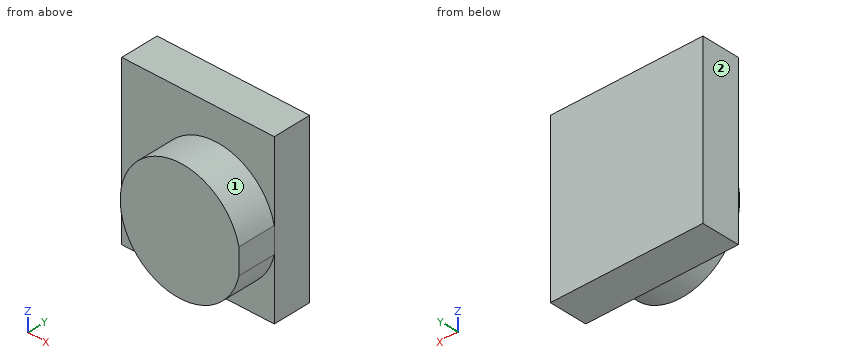
from build123d import *

# Parameters (mm, degrees)
F0_W     = 101.685505
F0_H     = 110.430561
F1_DEPTH = 25.4
F3_DEPTH = 25.4


with BuildPart() as f1:
    # F0 (on Front) → F1 (new body)
    with BuildSketch(Plane.XZ):
        with Locations((-2.378846, 5.691071)):
            Rectangle(F0_W, F0_H)
    extrude(amount=F1_DEPTH)

    # F2 (on face) → F3 (join)
    with BuildSketch(Plane.XZ.offset(25.4)):
        with BuildLine():
            Line((48.463907, -8.572468), (48.463907, 8.572468))
            ThreePointArc((48.463907, 8.572468), (-30.630272, 0), (48.463907, -8.572468))
        make_face()
    extrude(amount=F3_DEPTH)


solid = f1.part
The model under review builds one solid part; all positions refer to its coordinate system, in mm. Face numbers are marked on the shaded views. A direction names the side the tool comes from. Give positions to 0.01 mm unless a question says otherwise; leave off trailing zeros. Loops run counter-clockwise (first coordinate to the right, second up) from the corner with the lowest first, then second, coordinate; pieces in that order, holes last. Notation, with made-up numbers: (47, 0) -> (101, 0) arc R11 cw to (101, 9) -> close; hole circle Ø11 at (47, 31). An arc over 180 degrees is marked (long way). Put each result on its own line as item: value. Start each with the question number.
1. We need section C-C on y = -31.5. State the section outline as (x, z) points, then the cut area to 3 significant figures.
2. Wall thickness on probe 1 along Y at (x, z) = (43.5, 56); probe 2 along Z at (x, y) = (27, -41); probe 3 along X at (y, z) = (-28.5, 34.5): over which ranges is each line inside the solid? List them lowest first.
3. We need section B-B on x = 20. State the section outline as (y, z) points.
4. For the marked faces 1 and 2, list the 3-axis set-ups (+Z, -Z, +X, -X, +Y, -Y) from which the entire face can be reached by the end or side of a thin tool; tool diameter is ignored.
5. Clearance check with flat-ended pins moving along their axes: P1, Ø5, axis at y = -31.5, z = -37, coming from the -X side; P2, Ø3, axis at y = -35, z = -4.5, coming from the -X side; P3, Ø6, axis at x = 11, z = 47, coming from the -Y side. State where each tip first meets the part, or that it passes through.
6. We need section A-A on z = 0. State the section outline as (x, y) points.
7. We need section D-D on x = -25. State the section outline as (y, z) points, then the cut area to 3 significant figures.
Determined:
1. outline: (48.46, -8.57) -> (48.46, 8.57) arc R40.01 ccw (long way) to start
1. area: 5,020 mm^2
2. probe 1: -25.4 to 0
2. probe 2: -35.92 to 35.92
2. probe 3: -10.88 to 29.65
3. outline: (-50.8, -38.58) -> (-25.4, -38.58) -> (-25.4, -49.52) -> (0, -49.52) -> (0, 60.91) -> (-25.4, 60.91) -> (-25.4, 38.58) -> (-50.8, 38.58) -> close
4. face 1: -Y
4. face 2: +Z, -Z, -X, +Y, -Y
5. P1: x = -10.88
5. P2: x = -30.52
5. P3: y = -25.4
6. outline: (-53.22, -25.4) -> (-30.63, -25.4) -> (-30.63, -50.8) -> (48.46, -50.8) -> (48.46, 0) -> (-53.22, 0) -> close
7. outline: (-50.8, -20.47) -> (-25.4, -20.47) -> (-25.4, -49.52) -> (0, -49.52) -> (0, 60.91) -> (-25.4, 60.91) -> (-25.4, 20.47) -> (-50.8, 20.47) -> close
7. area: 3,840 mm^2
